Part model, mm, in its own coordinate system. Face numbers are marked on the shaded views. A direction names the side the tool comes from. Coordinates: 2 decimals unless noted, no trailing zeros. Loops run counter-clockwise (first coordinate to the right, second up) from the corner with the lowest first, then second, coordinate; pieces in that order, holes last. Notation, with made-up numbers: M 11.25,-25.75 L 48.25,-25.75 A29 ccw 48.25,11.25 Z; hole C 61,46 d9. An arc over 180 degrees is marked long. Use CSV: the item, a comma, the result in double quotes. Start each with the question number.
Autodesk Inventor part; units mm, degrees
ref_plane "YZ Plane" through (0, 0, 0) normal (1, 0, 0) x (0, 1, 0)
ref_plane "XZ Plane" through (0, 0, 0) normal (0, 1, 0) x (-1, 0, 0)
ref_plane "XY Plane" through (0, 0, 0) normal (0, 0, 1) x (1, 0, 0)
sketch "Sketch1" plane through (0, 0, 0) normal (0, 0, 1) x (1, 0, 0)
  line L0 (0, 52.5) -> (25.1, 52.5)
  line L1 (33.1, 32.75) -> (33.1, -32.75)
  line L2 (0, -48.25) -> (5.56, -48.25)
  line L3 (27, -30.7) -> (30.6, -30.7)
  line L4 (30.6, -30.7) -> (30.6, 30.7)
  line L5 (30.6, 30.7) -> (27, 30.7)
  line L6 (25.1, 48.35) -> (22.6, 48.35)
  arc A0 (-0.95, -49.45) -> (-0.95, -50.75) centre (-0.95, -50.1) ccw
  line L7 (-0.95, -49.45) -> (0, -49.45)
  line L8 (0, -49.45) -> (0, -48.25)
  line L9 (-0.95, -50.75) -> (0, -50.75)
  line L10 (0, -50.75) -> (0, -52.5)
  line L11 (0, -52.5) -> (25.1, -52.5)
  line L12 (25.1, -52.5) -> (25.1, -50)
  line L13 (25.1, -50) -> (29, -50)
  line L14 (29, -50) -> (29, -47.55)
  line L15 (29, -47.55) -> (31.5, -47.55)
  line L16 (31.5, -47.55) -> (31.5, -50)
  line L17 (31.5, -50) -> (33.1, -50)
  line L18 (25.1, 52.5) -> (25.1, 50)
  line L19 (25.1, 50) -> (29, 50)
  line L20 (29, 50) -> (29, 47.55)
  line L21 (29, 47.55) -> (31.5, 47.55)
  line L22 (31.5, 47.55) -> (31.5, 50)
  line L23 (31.5, 50) -> (33.1, 50)
  arc A1 (1.85, 49.45) -> (1.85, 50.95) centre (1.85, 50.2) ccw
  line L24 (0, 49.45) -> (0, 48.35)
  line L25 (0, 50.95) -> (0, 52.5)
  line L26 (1.85, 50.95) -> (0, 50.95)
  line L27 (1.85, 49.45) -> (0, 49.45)
  line L28 (27, 30.7) -> (27, 39.7)
  line L29 (27, 39.7) -> (25.1, 39.7)
  line L30 (25.1, 46.25) -> (25.1, 48.35)
  line L31 (27, -30.7) -> (27, -39.7)
  line L32 (27, -39.7) -> (25.1, -39.7)
  line L33 (25.1, -46.25) -> (25.1, -48.25)
  line L34 (-8.54, 0) -> (40.04, 0)
  line L35 (33.1, 50) -> (33.1, 45.6)
  line L36 (33.1, 45.6) -> (31.1, 45.6)
  line L37 (31.1, 45.6) -> (31.1, 37.6)
  line L38 (31.1, 37.6) -> (33.1, 37.6)
  line L39 (33.1, -37.6) -> (31.1, -37.6)
  line L40 (31.1, -37.6) -> (31.1, -45.6)
  line L41 (31.1, -45.6) -> (33.1, -45.6)
  line L42 (33.1, -45.6) -> (33.1, -50)
  line L43 (33.1, 37.6) -> (33.1, 35.75)
  line L44 (33.1, 35.75) -> (30.55, 34.25)
  line L45 (30.55, 34.25) -> (33.1, 32.75)
  line L46 (33.1, -32.75) -> (30.55, -34.25)
  line L47 (30.55, -34.25) -> (33.1, -35.75)
  line L48 (33.1, -35.75) -> (33.1, -37.6)
  line L49 (22.6, 48.35) -> (22.6, 50.2)
  line L50 (22.6, 50.2) -> (20.8, 50.2)
  line L51 (20.8, 50.2) -> (20.8, 48.35)
  line L52 (20.8, 48.35) -> (17.52, 48.35)
  line L53 (17.52, 48.35) -> (17.52, 50.2)
  line L54 (17.52, 50.2) -> (15.72, 50.2)
  line L55 (15.72, 50.2) -> (15.72, 48.35)
  line L56 (15.72, 48.35) -> (12.44, 48.35)
  line L57 (12.44, 48.35) -> (12.44, 50.2)
  line L58 (12.44, 50.2) -> (10.64, 50.2)
  line L59 (10.64, 50.2) -> (10.64, 48.35)
  line L60 (10.64, 48.35) -> (7.36, 48.35)
  line L61 (7.36, 48.35) -> (7.36, 50.2)
  line L62 (7.36, 50.2) -> (5.56, 50.2)
  line L63 (5.56, 50.2) -> (5.56, 48.35)
  line L64 (5.56, 48.35) -> (0, 48.35)
  line L65 (5.56, -48.25) -> (5.56, -50.2)
  line L66 (5.56, -50.2) -> (7.36, -50.2)
  line L67 (7.36, -50.2) -> (7.36, -48.25)
  line L68 (7.36, -48.25) -> (10.64, -48.25)
  line L69 (10.64, -48.25) -> (10.64, -50.2)
  line L70 (10.64, -50.2) -> (12.44, -50.2)
  line L71 (12.44, -50.2) -> (12.44, -48.25)
  line L72 (12.44, -48.25) -> (15.72, -48.25)
  line L73 (15.72, -48.25) -> (15.72, -50.2)
  line L74 (15.72, -50.2) -> (17.52, -50.2)
  line L75 (17.52, -50.2) -> (17.52, -48.25)
  line L76 (17.52, -48.25) -> (20.8, -48.25)
  line L77 (20.8, -48.25) -> (20.8, -50.2)
  line L78 (20.8, -50.2) -> (22.6, -50.2)
  line L79 (22.6, -50.2) -> (22.6, -48.25)
  line L80 (22.6, -48.25) -> (25.1, -48.25)
  line L81 (25.1, 42.65) -> (25.1, 39.7)
  line L82 (25.1, 42.65) -> (25.85, 42.65)
  line L83 (25.85, 42.65) -> (25.85, 41.8)
  line L84 (25.85, 41.8) -> (27.55, 41.8)
  line L85 (27.55, 41.8) -> (27.55, 42.65)
  line L86 (27.55, 42.65) -> (28.6, 42.65)
  line L87 (28.6, 42.65) -> (28.6, 46.25)
  line L88 (28.6, 46.25) -> (27.55, 46.25)
  line L89 (27.55, 46.25) -> (27.55, 47.1)
  line L90 (27.55, 47.1) -> (25.85, 47.1)
  line L91 (25.85, 47.1) -> (25.85, 46.25)
  line L92 (25.85, 46.25) -> (25.1, 46.25)
  line L93 (25.1, -46.25) -> (25.85, -46.25)
  line L94 (25.85, -46.25) -> (25.85, -47.1)
  line L95 (25.85, -47.1) -> (27.55, -47.1)
  line L96 (27.55, -47.1) -> (27.55, -46.25)
  line L97 (27.55, -46.25) -> (28.6, -46.25)
  line L98 (28.6, -46.25) -> (28.6, -42.65)
  line L99 (28.6, -42.65) -> (27.55, -42.65)
  line L100 (27.55, -42.65) -> (27.55, -41.8)
  line L101 (27.55, -41.8) -> (25.85, -41.8)
  line L102 (25.85, -41.8) -> (25.85, -42.65)
  line L103 (25.85, -42.65) -> (25.1, -42.65)
  line L104 (25.1, -42.65) -> (25.1, -39.7)
  point P0 (0, 0)
  dimension "d7" = 21.8
  dimension "d10" = 0.65
  dimension "d11" = 34.7
  dimension "d14" = 105
  dimension "d16" = 100
  dimension "d17" = 95.1
  dimension "d18" = 2.5
  dimension "d20" = 1.6
  dimension "d24" = 2.5
  dimension "d29" = 96.6
  dimension "d30" = 1.85
  dimension "d31" = 1.5
  dimension "d32" = 100.3
  dimension "d33" = 8
  dimension "d34" = 33.1
  dimension "d35" = 2.6
  dimension "d36" = 12.8
  dimension "d37" = 6.1
  dimension "d49" = 8
  dimension "d50" = 4.4
  dimension "d51" = 4.1
  dimension "d52" = 3
  dimension "d53" = 2.55
  dimension "d55" = 68.5
  dimension "d56" = 1.8
  dimension "d57" = 5.08
  dimension "d58" = 10.5
  dimension "d59" = 4.15
  dimension "d60" = 3.6
  dimension "d61" = 0.75
  dimension "d62" = 1.7
  dimension "d63" = 3.5
  dimension "d64" = 5.3
  dimension "d65" = 94.2
extrude "Extrusion1" add sketch "Sketch1" along normal blind 167.2
sketch "Sketch2" plane through (0, 0, 167.2) normal (0, 0, 1) x (1, 0, 0)
  line L0 (33.1, -50) -> (33.1, 50)
  line L1 (-8.54, 0) -> (40.04, 0)
  point P0 (0, 0)
  point P1 (30.55, 34.25)
  point P2 (30.55, -34.25)
  dimension "d40" = 2.55
  dimension "d41" = 68.5
hole "Hole1" at (30.55, -34.25, 167.2) at (30.55, 34.25, 167.2) direction (0, 0, -1) diameter 3 end through all
properties part number "Fischer HB"
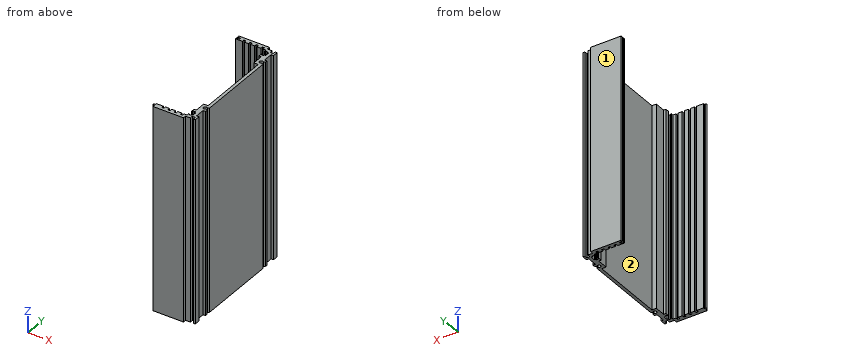
1. Pin check, flat tips, straight feed: pin 1 (1 mm diameter, centred on y = -6.5, z = 50, fed in from -X); pin 2 (1.5 mm diameter, centred on y = -37.5, z = 72, fed in from -X); pin 3 (0.6 mm diameter, centred on x = 32.5, z = 70.5, fed in from -Y). Stop position of each tip, or through.
2. Wall check: probe 1 along Y at (x, z) = (30.55, 74.5); probe 2 along Y at (x, z) = (14, 7.5); probe 3 along Y at (x, z) = (30, 60.5). Give the ranges that are in metal, low to high.
3. Slice it at A-A, the plane y = 19. List the corners of the cut face in (x, z), and give its area (3 significant figures).
4. Tool access for the marked faces 1 and 2: list every direction of +Z, -Z, +X, -X, +Y, -Y with a clear straight run to the whole face (end or side of a thin tool).
Found:
1,pin 1,"x = 30.6"
1,pin 2,"x = 27"
1,pin 3,"y = -50"
2,probe 1,"-47.55 to -35.75, -32.75 to -30.7, 30.7 to 32.75, 35.75 to 47.55"
2,probe 2,"-52.5 to -48.25, 48.35 to 52.5"
2,probe 3,"-47.55 to -35.65, -32.85 to -30.7, 30.7 to 32.85, 35.65 to 47.55"
3,outline,"M 30.6,0 L 33.1,0 L 33.1,167.2 L 30.6,167.2 Z"
3,area,"418 mm^2"
4,face 1,"+Z, -Z, +X, -X, +Y"
4,face 2,"+Z, -Z, -X"
